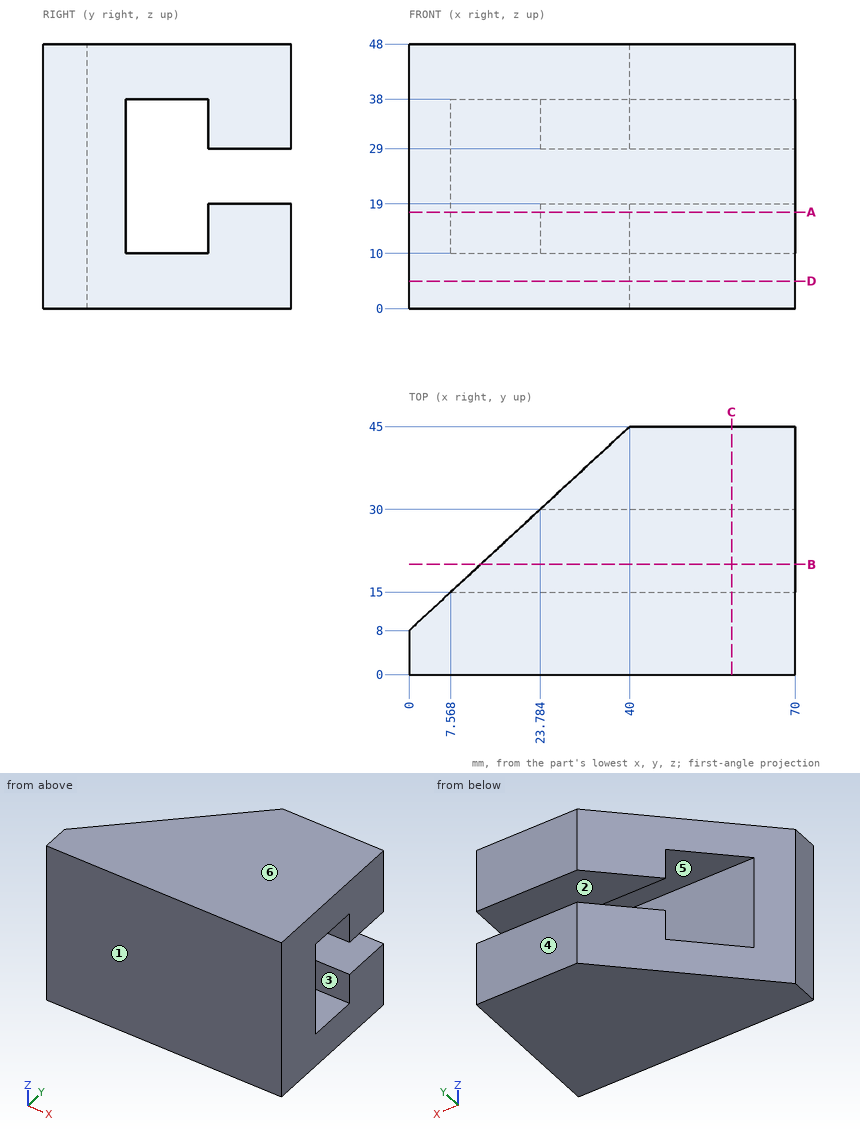
Can you work these out from the drawing? Everything is in mm from the part's minimum corner. A direction names the side the tool comes from. Give positions to 0.01 mm unless a question says otherwise; leave off trailing zeros. Loops run counter-clockwise (first coordinate to the right, second up) from the corner with the lowest first, then second, coordinate; pieces in that order, holes last. Notation, with made-up numbers: (-26.75, 33) - (10.25, 33) arc R25 cw to (10.25, 72) - close; hole circle Ø7 at (26, -4.5). An arc over 180 degrees is marked (long way). Answer as a JSON object with one key per item and string values.
Q1. If I drill on L1, parallel to Z at x = 51, y = 24.5; L2, parallel to Z at x = 39, y = 39; L3, parallel to Y at x = 53, z = 37.5, over which ranges is the centre line in solid material (lowest first)?
Geometry says:
{"L1": "0 to 10, 38 to 48", "L2": "0 to 19, 29 to 48", "L3": "0 to 15, 30 to 45"}
Q2. Imagine slicing it at B-B on y = 20. Write out the boundary of the cut face in (x, z).
Geometry says:
{"outline": "(12.97, 0) - (70, 0) - (70, 10) - (12.97, 10) - close; (12.97, 38) - (70, 38) - (70, 48) - (12.97, 48) - close"}
Q3. Imagine slicing it at A-A on z = 17.5. Write out the boundary of the cut face in (x, y).
Geometry says:
{"outline": "(0, 0) - (70, 0) - (70, 15) - (7.57, 15) - (0, 8) - close; (23.78, 30) - (70, 30) - (70, 45) - (40, 45) - close"}
Q4. Which directions (+Z, -Z, +X, -X, +Y, -Y) give clear straight access to the entire face, cutting with the end or side of a thin tool? Please do the marked faces 1, 2 and 3.
Geometry says:
{"face 1": "+Z, -Z, +X, -X, -Y", "face 2": "+X, -X, +Y", "face 3": "+X, -X"}
Q5. Imagine slicing it at C-C on x = 58.5. Write out the boundary of the cut face in (y, z), plus the area to 3 significant figures.
Geometry says:
{"outline": "(0, 0) - (45, 0) - (45, 19) - (30, 19) - (30, 10) - (15, 10) - (15, 38) - (30, 38) - (30, 29) - (45, 29) - (45, 48) - (0, 48) - close", "area": "1,590 mm²"}
Q6. Imagine slicing it at D-D on z = 5. Write out the boundary of the cut face in (x, y), plus the area to 3 significant figures.
Geometry says:
{"outline": "(0, 0) - (70, 0) - (70, 45) - (40, 45) - (0, 8) - close", "area": "2,410 mm²"}
Q7. If we mould it in two halves opening along Y, with no side actions, what happens to the marked faces 4, 5 and 6? For each: pulls with the +Y half, pulls with the -Y half, needs draft (parallel to the pull), parting line crosses it, or undercut.
Geometry says:
{"face 4": "pulls with the +Y half", "face 5": "undercut", "face 6": "needs draft"}
